Study the drawing (mm; zero at the part's minimum x, y, z) and answer. Round coordinates to 2 decimals unless told otherwise and drop trailing zeros. Loops run counter-clockwise (first coordinate to the right, second up) from the corner with the lowest first, then second, coordinate; pieces in that order, holes last. Notation, with made-up numbers: (-34.75, 36) -> (-8.75, 36) arc R16 ccw to (-8.75, 52) -> close; hole circle Ø10 at (50, 57.5). An arc over 180 degrees is marked (long way). Use one line per item in the form item = value.
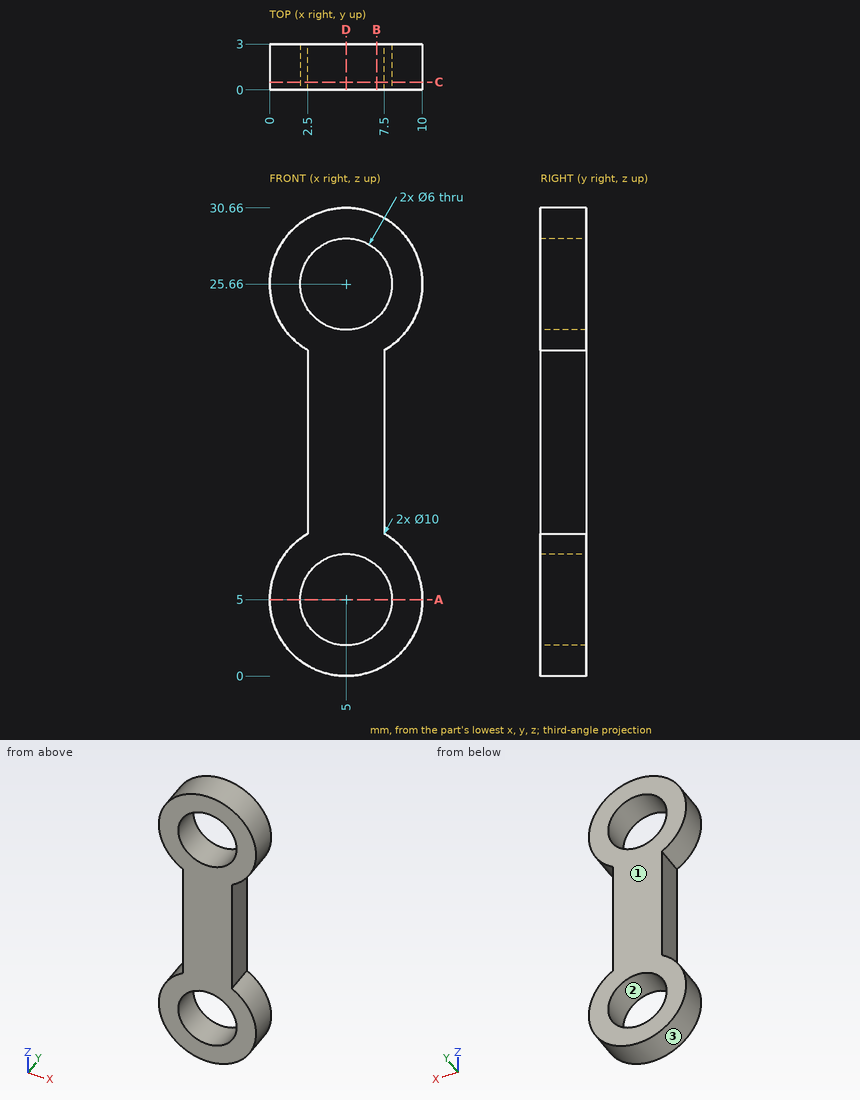
(1) Given P1, Ø5.5, axis at x = 5, z = 5, coming from the -Y side, flat-ended and moving along its own axis, determine where the tip first touches the part or whether it passes through.
Completed:
P1 = through
(2) Find section A-A, the plane z = 5. Write down the section's boundary in (x, y), then the cut area to 3 significant figures.
Completed:
outline = (0, 0) -> (2, 0) -> (2, 3) -> (0, 3) -> close; (8, 0) -> (10, 0) -> (10, 3) -> (8, 3) -> close
area = 12.0 mm2
(3) Find section D-D, the plane x = 5. Write down the section's boundary in (y, z), then the cut area to 3 significant figures.
Completed:
outline = (0, 0) -> (3, 0) -> (3, 2) -> (0, 2) -> close; (0, 8) -> (3, 8) -> (3, 22.66) -> (0, 22.66) -> close; (0, 28.66) -> (3, 28.66) -> (3, 30.66) -> (0, 30.66) -> close
area = 56.0 mm2
(4) Find section C-C, the plane y = 0.5. Write down the section's boundary in (x, z), then the cut area to 3 significant figures.
Completed:
outline = (2.5, 9.33) arc R5 ccw (long way) to (7.5, 9.33) -> (7.5, 21.33) arc R5 ccw (long way) to (2.5, 21.33) -> close; hole circle Ø6 at (5, 5); hole circle Ø6 at (5, 25.66)
area = 156 mm2
(5) Consider L1, parallel to X at y = 1.75, z = 6; L2, parallel to X at y = 1.65, z = 14; L3, parallel to Z at x = 9.5, y = 0.8. Determine where each line is inside the solid, lowest interval first.
Completed:
L1 = 0.1 to 2.17, 7.83 to 9.9
L2 = 2.5 to 7.5
L3 = 2.82 to 7.18, 23.48 to 27.84
(6) For a pull along X with two mould halves and no side action, classify the marked faces 1, 2 and 3 as +X half, -X half, draft (parallel to the pull), parting line (faces both ways), or undercut.
Completed:
face_1 = draft
face_2 = undercut
face_3 = parting line
(7) Find section B-B, the plane x = 7. Write down the section's boundary in (y, z).
Completed:
outline = (0, 0.42) -> (3, 0.42) -> (3, 2.76) -> (0, 2.76) -> close; (0, 7.24) -> (3, 7.24) -> (3, 23.42) -> (0, 23.42) -> close; (0, 27.9) -> (3, 27.9) -> (3, 30.24) -> (0, 30.24) -> close
